Autodesk Fusion 360 part; units mm, degrees
sketch "Esquisse1" plane through (0, 0, 0) normal (0, 0, 1) x (1, 0, 0)
  line L0 (100, 78) -> (-100, 78)
  line L1 (-100, 78) -> (-100, -78)
  line L2 (-100, -78) -> (100, -78)
  line L3 (100, -78) -> (100, 78)
  line L4 (100, 78) -> (-100, -78) construction
  line L5 (-100, 78) -> (100, -78) construction
  line L6 (103, -75) -> (-103, -75)
  line L7 (-103, -75) -> (-103, 75)
  line L8 (-103, 75) -> (103, 75)
  line L9 (103, 75) -> (103, -75)
  line L10 (103, -75) -> (-103, 75) construction
  line L11 (-103, -75) -> (103, 75) construction
  dimension "d1" = 200
  dimension "d2" = 206
  dimension "d3" = 150
  dimension "d4" = 156
extrude "Extrusion1" add sketch "Esquisse1" along normal blind 3
sketch "Esquisse4" plane through (0, 0, 3) normal (0, 0, 1) x (-1, 0, 0)
  line L0 (-100, -75) -> (-100, -78)
  line L1 (-100, -78) -> (100, -78)
  line L2 (100, -78) -> (100, -75)
  line L3 (100, -75) -> (103, -75)
  line L4 (103, -75) -> (103, 75)
  line L5 (103, 75) -> (100, 75)
  line L6 (100, 75) -> (100, 78)
  line L7 (100, 78) -> (-100, 78)
  line L8 (-100, 78) -> (-100, 75)
  line L9 (-100, 75) -> (-103, 75)
  line L10 (-103, 75) -> (-103, -75)
  line L11 (-103, -75) -> (-100, -75)
  line L12 (-2.5, 49) -> (67, 49)
  line L13 (67, 49) -> (67, -49)
  line L14 (67, -49) -> (-2.5, -49)
  line L15 (-2.5, -49) -> (-2.5, 49)
  line L16 (-2.5, 49) -> (67, -49) construction
  line L17 (67, 49) -> (-2.5, -49) construction
  line L18 (-48, 48) -> (-20.5, 48)
  line L19 (-20.5, 48) -> (-20.5, -27)
  line L20 (-20.5, -27) -> (-48, -27)
  line L21 (-48, -27) -> (-48, 48)
  line L22 (-48, 48) -> (-20.5, -27) construction
  line L23 (-20.5, 48) -> (-48, -27) construction
  circle A0 centre (67, -49) radius 1.7
  circle A1 centre (-2.5, -49) radius 1.7
  circle A2 centre (-20.5, -27) radius 1.6
  circle A3 centre (-48, -27) radius 1.6
  circle A4 centre (-20.5, 48) radius 1.6
  circle A5 centre (-48, 48) radius 1.6
  line L24 (67, -49) -> (-2.5, -49)
  line L25 (-2.5, -49) -> (-2.5, 38)
  line L26 (-2.5, 38) -> (67, 38)
  line L27 (67, 38) -> (67, -49)
  circle A6 centre (67, 49) radius 1.7
  circle A7 centre (-2.5, 38) radius 1.7
  line L28 (-83, -15) -> (-83, 15)
  line L29 (-68, -20) -> (-78, -20)
  arc A8 (-68, -20) -> (-63, -15) centre (-68, -15) ccw
  line L30 (-63, 20) -> (-83, -20) construction
  line L31 (-78, 20) -> (-68, 20)
  arc A9 (-63, 15) -> (-68, 20) centre (-68, 15) ccw
  arc A10 (-78, 20) -> (-83, 15) centre (-78, 15) ccw
  line L32 (-83, 20) -> (-63, -20) construction
  line L33 (-63, 15) -> (-63, -15)
  arc A11 (-83, -15) -> (-78, -20) centre (-78, -15) ccw
  point P0 (32.25, 0)
  point P1 (-34.25, 10.5)
  point P2 (-73, 0)
  dimension "d26" = 69.5
  dimension "d27" = 98
  dimension "d28" = 27.5
  dimension "d29" = 75
  dimension "d30" = 18
  dimension "d31" = 3.4
  dimension "d34" = 3.4
  dimension "d35" = 3.2
  dimension "d36" = 3.2
  dimension "d37" = 3.2
  dimension "d38" = 3.2
  dimension "d39" = 87
  dimension "d43" = 3.4
  dimension "d44" = 3.4
  dimension "d45" = 5
  dimension "d46" = 20
  dimension "d47" = 15
  dimension "d48" = 20
  dimension "d49" = 40
  dimension "d50" = 29
  dimension "d51" = 58
  dimension "d52" = 30
extrude "Extrusion4" cut sketch "Esquisse4" against normal blind 3 contours L12 L13 A6 | L12 L13 A6 | L15 L26 A7 | L15 L25 A7 | L15 L25 L26 A7 | L14 L15 A1 L24 L25 | L14 L15 A1 L24 L25 | L13 L14 A0 L24 L27 | L13 L14 A0 L24 L27 | L18 L21 A5 | L18 L21 A5 | L18 L19 A4 | L18 L19 A4 | L20 L21 A3 | L20 L21 A3 | L19 L20 A2 | L19 L20 A2 | L28 L29 A8 L31 A9 A10 L33 A11
equation "d2 = d1 + ( 2 * 3 ) * 1 mm"
equation "d4 = d3 + ( 2 * 3 ) * 1 mm"
CAD build for the part. Positions are in the model's coordinates, mm. A direction names the side the tool comes from. Give positions to 0.01 mm unless a question says otherwise; leave off trailing zeros. Order: outer loops, then holes, each group sorted by start corner. A loop starts at its lowest first (then second) coordinate and runs counter-clockwise, first axis right, second up.
(1) Drill centre lines: L1, parallel to Y at x = 2.5, z = 1.7; L2, parallel to Y at x = 20.5, z = 2.3; L3, parallel to X at y = -15.5, z = 1. Where is each one in solid material? Low to high.
(2) Saw through at B-B, the plane y = -5. Give the cut face in (x, z), then the cut area to 3 significant figures.
(3) Flat gauge pins, fed straight in: pin 1 (5.5 mm diameter, centred on x = -67, y = 49, fed in from +Z); pin 2 (1.5 mm diameter, centred on x = -101, z = 2, fed in from -Y); pin 3 (1.5 mm diameter, centred on y = 76.5, z = 1.5, fed in from -X). Where does each tip first touch, or does it go through?
(4) Tool access for faces 1 (the cylindrical face through (64, -18, 2)), 2 (the flat face through (-1, 1, 0)): list every direction of +Z, -Z, +X, -X, +Y, -Y with a clear straight run to the whole face (end or side of a thin tool).
(5) Saw through at A-A, the plane z = 0.95. State how many separate pieces and enclosed holes the cut face has, then the cut area to 3 significant figures.
(6) Mould opens along Y. For faces 3 (the cylindrical face through (82, 18, 2)), 4 (the flat face through (-1, 1, 3)) say: released by +Y, released by -Y, zero draft, split by the parting line, or undercut.
Results found:
1. L1: y = -78 to -39.7, -36.3 to 47.3, 50.7 to 78
1. L2: y = -78 to -49.6, -46.4 to 25.4, 28.6 to 78
1. L3: x = -103 to 63.03, 82.97 to 103
2. outline: (-103, 0) - (63, 0) - (63, 3) - (-103, 3) - close; (83, 0) - (103, 0) - (103, 3) - (83, 3) - close
2. area: 558 mm2
3. pin 1: stops at z = 3
3. pin 2: stops at y = -75
3. pin 3: stops at x = -100
4. face 1: +Z, -Z
4. face 2: -Z, +X, -X, +Y, -Y
5. separate pieces: 1
5. enclosed holes: 9
5. area: 31,300 mm2
6. face 3: undercut
6. face 4: zero draft
